Here's how the part is built. I have some questions about the finished solid (model axes, mm). Coordinates: 2 decimals unless noted, no trailing zeros. Write each loop counter-clockwise with the first axis right and the second up, starting at its lowest first coordinate (ties: lowest second). Pieces come first, ordered by that corner, then holes. Notation, with made-up numbers: (66, 5) -> (88, 5) arc R21 ccw to (88, 20) -> close; hole circle Ø11 at (16.25, 48.25). An arc over 180 degrees is marked (long way). Put each result on its own line as item: value.
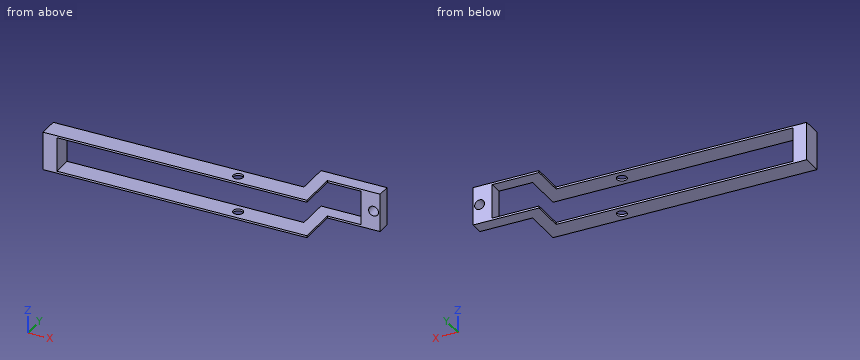
```python
from build123d import *

# Parameters (mm, degrees)
SKETCH1_R           = 4.7625
BOSS_EXTRUDE1_DEPTH = 36.83
SKETCH2_W           = 273.05
SKETCH2_H           = 33.02
CUT_EXTRUDE1_DEPTH  = 312.191466625
SKETCH4_R           = 4.7625
CUT_EXTRUDE3_DEPTH  = 312.191466625


with BuildPart() as part:
    # Sketch1 → Boss-Extrude1 (new body)
    with BuildSketch(Plane.XY):
        Polygon((304.8, 50.8), (304.8, 38.1), (254, 38.1), (254, 0), (0, 0), (0, 19.05), (241.3, 19.05), (241.3, 50.8), align=None)
        with Locations((182.88, 9.525)):
            Circle(SKETCH1_R, mode=Mode.SUBTRACT)
    extrude(amount=BOSS_EXTRUDE1_DEPTH)

    # Sketch2 → Cut-Extrude1 (cut, through all)
    with BuildSketch(Plane.XZ):
        with Locations((149.876052358, 18.415)):
            Rectangle(SKETCH2_W, SKETCH2_H)
    extrude(amount=-CUT_EXTRUDE1_DEPTH, mode=Mode.SUBTRACT)

    # Sketch4 → Cut-Extrude3 (cut, through all)
    with BuildSketch(Plane(origin=(0, 50.8, 0), x_dir=(1, 0, 0), z_dir=(0, 1, 0))):
        with Locations(Location((298.45, -18.415, 0), (0, 0, 270))):
            Circle(SKETCH4_R)
    extrude(amount=-CUT_EXTRUDE3_DEPTH, mode=Mode.SUBTRACT)


solid = part.part
```
Item 1: For P1, Ø1, axis at y = 37, z = 1, coming from the -X side; P2, Ø5.5, axis at x = 182.88, y = 9.525, coming from the +Z side; P3, Ø3, axis at y = 16.5, z = 21.5, coming from the +X side; P4, Ø12, axis at y = 45, z = 25, coming from the -X side, each with a flat end and sliding along its axis, tell me the tip position at first contact or that it passes through.
Output:
P1: stops at x = 241.3
P2: passes through
P3: stops at x = 13.35
P4: stops at x = 286.4
Item 2: Please list where these lines run through material, in increasing order: line 1 along Z through (x, y) = (286, 44) (3 decimals); line 2 along Z through (x, y) = (298.45, 48); line 3 along X through (y, z) = (15, 7.5). Write a range as from..to.
Output:
line 1: z = 0..1.905, 34.925..36.83
line 2: z = 0..13.65, 23.18..36.83
line 3: x = 0..13.35
Item 3: Imagine slicing it at D-D on z = 28.5. Write out the boundary of the cut face in (x, y).
Output:
outline: (0, 0) -> (13.35, 0) -> (13.35, 19.05) -> (0, 19.05) -> close; (286.4, 38.1) -> (304.8, 38.1) -> (304.8, 50.8) -> (286.4, 50.8) -> close
Item 4: Imagine slicing it at C-C on x = 103. Write out the boundary of the cut face in (y, z) (3 decimals), then the cut area to 3 significant figures.
Output:
outline: (0, 0) -> (19.05, 0) -> (19.05, 1.905) -> (0, 1.905) -> close; (0, 34.925) -> (19.05, 34.925) -> (19.05, 36.83) -> (0, 36.83) -> close
area: 72.6 mm²
Item 5: Imagine slicing it at A-A on x = 182.88. State how many separate pieces and enclosed holes the cut face has, then the cut area to 3 significant figures.
Output:
separate pieces: 4
enclosed holes: 0
area: 36.3 mm²
